```python
from build123d import *

# Parameters (mm, degrees)
F0_R       = 5.25
F1_DEPTH   = 20
F2_W       = 20.2225241501
F2_H       = 1
F3_DEPTH   = 20.001
F4_R       = 2.625
F5_DEPTH   = 5.001
F6_SIZE2   = 8
F6_SIZE    = 4
F7_SIZE2   = 4
F7_SIZE    = 8
F7_2_SIZE2 = 4
F7_2_SIZE  = 8
F8_R       = 2


with BuildPart() as f1:
    # F0 (on Top) → F1 (new body)
    with BuildSketch(Plane.XY):
        with BuildLine():
            Line((-10.2225241501, 5), (-20.2225241501, 5))
            Line((-20.2225241501, 5), (-20.2225241501, 0))
            Line((-20.2225241501, 0), (20.2225241501, 0))
            Line((20.2225241501, 0), (20.2225241501, 5))
            Line((20.2225241501, 5), (10.2225241501, 5))
            ThreePointArc((10.2225241501, 5), (8.180287213, 5.8024403779), (7.2305658623, 7.7804878049))
            ThreePointArc((7.2305658623, 7.7804878049), (0, 14.5), (-7.2305658623, 7.7804878049))
            ThreePointArc((-7.2305658623, 7.7804878049), (-8.180287213, 5.8024403779), (-10.2225241501, 5))
        make_face()
        with Locations((0, 7.25)):
            Circle(F0_R, mode=Mode.SUBTRACT)
    extrude(amount=F1_DEPTH)

    # F2 (on face) → F3 (cut, through all)
    with BuildSketch(Plane.XY.offset(20)):
        with Locations((-10.1112620751, 2.5)):
            Rectangle(F2_W, F2_H)
    extrude(amount=-F3_DEPTH, mode=Mode.SUBTRACT)

    # F4 (on face) → F5 (cut, through all)
    with BuildSketch(Plane(origin=(0, 5, 0), x_dir=(-1, 0, 0), z_dir=(0, 1, 0))):
        with Locations((-15.2225241501, 10)):
            Circle(F4_R)
        with Locations((15.2225241501, 10)):
            Circle(F4_R)
    extrude(amount=-F5_DEPTH, mode=Mode.SUBTRACT)

    # F6
    f6_edges = [f1.edges().sort_by_distance(p)[0] for p in [
        (-20.222524, 1, 20),
        (-20.222524, 4, 20),
        (20.222524, 2.5, 20),
        (-20.222524, 1, 0),
    ]]
    chamfer(f6_edges, length=F6_SIZE, length2=F6_SIZE2)

    # F7
    f7_edges = [f1.edges().sort_by_distance(p)[0] for p in [
        (20.222524, 2.5, 0),
    ]]
    f7_side = f1.faces().sort_by_distance((20.222524, 2.5, 6))[0]
    chamfer(f7_edges, length=F7_SIZE, length2=F7_SIZE2, reference=f7_side)

    # F7#2
    f7_2_edges = [f1.edges().sort_by_distance(p)[0] for p in [
        (-20.222524, 4, 0),
    ]]
    f7_2_side = f1.faces().sort_by_distance((-20.222524, 4, 6))[0]
    chamfer(f7_2_edges, length=F7_2_SIZE, length2=F7_2_SIZE2, reference=f7_2_side)

    # F8
    f8_edges = [f1.edges().sort_by_distance(p)[0] for p in [
        (-3.082207, 3, 10),
    ]]
    fillet(f8_edges, radius=F8_R)


solid = f1.part
```
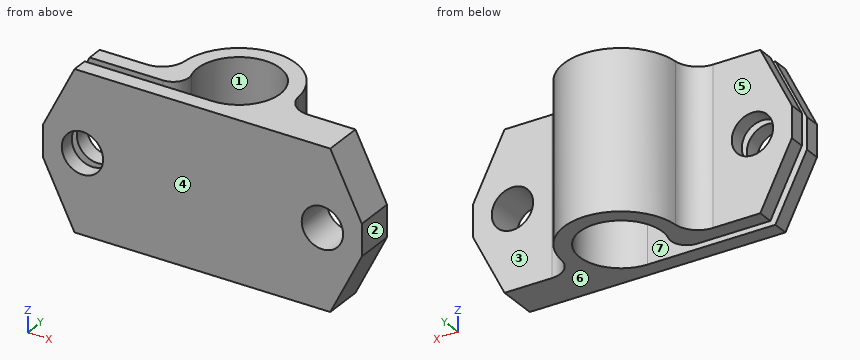
Model file for the job. Use its own axes, mm. Face numbers are marked on the shaded views. A direction names the side the tool comes from. Coordinates: 2 decimals unless noted, no trailing zeros. Loops run counter-clockwise (first coordinate to the right, second up) from the corner with the lowest first, then second, coordinate; pieces in that order, holes last. Notation, with made-up numbers: (71.5, 17.5) - (97.5, 17.5) arc R36 ccw to (97.5, 53.5) - close; hole circle Ø2 at (-37, -0.75). An arc over 180 degrees is marked (long way). Answer as a JSON object with one key per item and string values. Group by question number.
(1) Cut at C-C (z = 10). Give the cut face in (x, y), then the cut area to 3 significant figures.
(2) Cut at A-A (y = 1.5). Give the cut face in (x, z) (3 decimals), then the cut area to 3 significant figures.
(3) Cut at D-D (y = 9). Give the cut face in (x, z), then the cut area to 3 significant figures.
(4) Probe line 1 along Y through (x, z) = (0, 5.75); line 2 along X through (y, z) = (1.5, 11); line 3 along Y through (x, z) = (-10.5, 8). List the from-to ranges inside material, lowest first.
(5) Cut at B-B (x = -8.5). Give the cut face in (y, z), then the cut area to 3 significant figures.
(6) Tool access for the marked faces 5, 6 and 7: list every direction of +Z, -Z, +X, -X, +Y, -Y with a clear straight run to the whole face (end or side of a thin tool).
(7) Two-plate mould, pull along Y, no slides. Class the marked faces 1, 2, 3 and 4: released by +Y, released by -Y, zero draft, split by the parting line, or undercut.
(8) Flat gauge pins, fed straight in: pin 1 (11 mm diameter, centred on x = 14, z = 11.5, fed in from +Y); pin 2 (11 mm diameter, centred on x = -17.5, z = 7.5, fed in from +Y); pin 3 (2 mm diameter, centred on y = 12, z = 3.5, fed in from -X). Where does each tip first touch, or does it go through?
Geometry says:
{
 "1": {"outline": "(-20.22, 0) - (-17.85, 0) - (-17.85, 2) - (-20.22, 2) - close; (-20.22, 3) - (-17.85, 3) - (-17.85, 5) - (-20.22, 5) - close; (-12.6, 0) - (12.6, 0) - (12.6, 5) - (10.22, 5) arc R3 cw to (7.23, 7.78) arc R7.25 ccw to (-7.23, 7.78) arc R3 cw to (-10.22, 5) - (-12.6, 5) - (-12.6, 3) - (-6.89, 3) arc R2 ccw to (-4.99, 5.62) arc R5.25 cw (long way) to (0, 2) - (-12.6, 2) - close; (17.85, 0) - (20.22, 0) - (20.22, 5) - (17.85, 5) - close", "area": "167 mm^2"},
 "2": {"outline": "(-20.223, 8) - (-16.223, 0) - (16.223, 0) - (20.223, 8) - (20.223, 12) - (16.223, 20) - (-16.223, 20) - (-20.223, 12) - close; hole circle Ø5.25 at (-15.223, 10); hole circle Ø5.25 at (15.223, 10)", "area": "702 mm^2"},
 "3": {"outline": "(-7.04, 0) - (-4.95, 0) - (-4.95, 20) - (-7.04, 20) - close; (4.95, 0) - (7.04, 0) - (7.04, 20) - (4.95, 20) - close", "area": "83.4 mm^2"},
 "4": {"line 1": "y = 0 to 2, 12.5 to 14.5", "line 2": "x = -20.22 to -17.65, -12.8 to 12.8, 17.65 to 20.22", "line 3": "y = 0 to 2, 3 to 5"},
 "5": {"outline": "(0, 0) - (2, 0) - (2, 20) - (0, 20) - close; (3, 0) - (5.54, 0) - (5.54, 20) - (3, 20) - close", "area": "90.9 mm^2"},
 "6": {"face 5": "+Z, -Z, -X, +Y", "face 6": "-Z, +X, -X, +Y, -Y", "face 7": "+Z, -Z, -X"},
 "7": {"face 1": "undercut", "face 2": "zero draft", "face 3": "released by +Y", "face 4": "released by -Y"},
 "8": {"pin 1": "stops at y = 5.54", "pin 2": "stops at y = 5", "pin 3": "stops at x = -6.2"}
}
